Check sheet for the modelled part. Datum: model origin and axes. Units: mm. A direction names the side the tool comes from. Round coordinates to 2 decimals unless told otherwise and drop trailing zeros. Write each loop counter-clockwise with the first axis right and the second up, starting at its lowest first coordinate (ties: lowest second). Pieces come first, ordered by that corner, then holes. Notation, with made-up numbers: M -12,20 L -7,20 A30 ccw -7,56 Z; hole C 40,8 d8. An arc over 180 degrees is marked long. Answer in a Markdown table with one row per item.
```python
from build123d import *

# Parameters (mm, degrees)
SKETCH1_W           = 180
SKETCH1_H           = 140
BOSS_EXTRUDE1_DEPTH = 5.588
SKETCH3_R           = 2.65
CUT_EXTRUDE2_DEPTH  = 229.103541717
BOSS_EXTRUDE2_DEPTH = 5.588
SKETCH5_R           = 12.5
CUT_EXTRUDE3_DEPTH  = 246.465813799
SKETCH6_R           = 1.65
CUT_EXTRUDE4_DEPTH  = 246.465813799
SKETCH7_W           = 150
SKETCH7_H           = 42
BOSS_EXTRUDE3_DEPTH = 5.588
SKETCH2_R           = 2.15
CUT_EXTRUDE1_DEPTH  = 246.465813799
FILLET1_R           = 4


with BuildPart() as part:
    # Sketch1 → Boss-Extrude1 (new body)
    with BuildSketch(Plane(origin=(0, 0, 0), x_dir=(1, 0, 0), z_dir=(0, 1, 0))):
        with Locations((90, 70)):
            Rectangle(SKETCH1_W, SKETCH1_H)
    extrude(amount=BOSS_EXTRUDE1_DEPTH)

    # Sketch3 → Cut-Extrude2 (cut, through all)
    with BuildSketch(Plane(origin=(0, 5.588, 0), x_dir=(1, 0, 0), z_dir=(0, 1, 0))):
        with Locations(Location((90, 130, 0), (0, 0, 270))):
            Circle(SKETCH3_R)
        with Locations(Location((110, 130, 0), (0, 0, 270))):
            Circle(SKETCH3_R)
        with Locations(Location((130, 130, 0), (0, 0, 270))):
            Circle(SKETCH3_R)
        with Locations(Location((170, 130, 0), (0, 0, 270))):
            Circle(SKETCH3_R)
        with Locations(Location((30, 130, 0), (0, 0, 90))):
            Circle(SKETCH3_R)
        with Locations(Location((150, 130, 0), (0, 0, 270))):
            Circle(SKETCH3_R)
        with Locations(Location((10, 130, 0), (0, 0, 90))):
            Circle(SKETCH3_R)
        with Locations(Location((50, 130, 0), (0, 0, 90))):
            Circle(SKETCH3_R)
        with Locations(Location((70, 130, 0), (0, 0, 90))):
            Circle(SKETCH3_R)
        with Locations(Location((70, 10, 0), (0, 0, 270))):
            Circle(SKETCH3_R)
        with Locations(Location((50, 10, 0), (0, 0, 270))):
            Circle(SKETCH3_R)
        with Locations(Location((10, 10, 0), (0, 0, 270))):
            Circle(SKETCH3_R)
        with Locations(Location((150, 10, 0), (0, 0, 90))):
            Circle(SKETCH3_R)
        with Locations(Location((30, 10, 0), (0, 0, 270))):
            Circle(SKETCH3_R)
        with Locations(Location((170, 10, 0), (0, 0, 90))):
            Circle(SKETCH3_R)
        with Locations(Location((130, 10, 0), (0, 0, 90))):
            Circle(SKETCH3_R)
        with Locations(Location((110, 10, 0), (0, 0, 90))):
            Circle(SKETCH3_R)
        with Locations(Location((90, 10, 0), (0, 0, 90))):
            Circle(SKETCH3_R)
    extrude(amount=-CUT_EXTRUDE2_DEPTH, mode=Mode.SUBTRACT)

    # Sketch4 → Boss-Extrude2 (add, through all)
    with BuildSketch(Plane(origin=(0, 5.588, 0), x_dir=(1, 0, 0), z_dir=(0, 1, 0))):
        with BuildLine():
            Line((160, 140), (141.293647591, 140))
            ThreePointArc((141.293647591, 140), (135, 163.3), (128.706352409, 140))
            Line((128.706352409, 140), (110, 140))
            Line((110, 140), (110, 166.8))
            Line((110, 166.8), (160, 166.8))
            Line((160, 166.8), (160, 140))
        make_face()
    extrude(amount=-BOSS_EXTRUDE2_DEPTH)

    # Sketch5 → Cut-Extrude3 (cut, through all)
    with BuildSketch(Plane(origin=(0, 5.588, 0), x_dir=(1, 0, 0), z_dir=(0, 1, 0))):
        with Locations(Location((135, 150.8, 0), (0, 0, 270))):
            Circle(SKETCH5_R)
    extrude(amount=-CUT_EXTRUDE3_DEPTH, mode=Mode.SUBTRACT)

    # Sketch6 → Cut-Extrude4 (cut, through all)
    with BuildSketch(Plane(origin=(0, 5.588, 0), x_dir=(1, 0, 0), z_dir=(0, 1, 0))):
        with Locations(Location((115, 162.8, 0), (0, 0, 270))):
            Circle(SKETCH6_R)
        with Locations(Location((155, 162.8, 0), (0, 0, 270))):
            Circle(SKETCH6_R)
        with Locations(Location((155, 143.8, 0), (0, 0, 270))):
            Circle(SKETCH6_R)
        with Locations(Location((115, 143.8, 0), (0, 0, 270))):
            Circle(SKETCH6_R)
    extrude(amount=-CUT_EXTRUDE4_DEPTH, mode=Mode.SUBTRACT)

    # Sketch7 → Boss-Extrude3 (add, through all)
    with BuildSketch(Plane(origin=(0, 5.588, 0), x_dir=(1, 0, 0), z_dir=(0, 1, 0))):
        with Locations((-75, 70)):
            Rectangle(SKETCH7_W, SKETCH7_H)
    extrude(amount=-BOSS_EXTRUDE3_DEPTH)

    # Sketch2 → Cut-Extrude1 (cut, through all)
    with BuildSketch(Plane(origin=(0, 5.588, 0), x_dir=(1, 0, 0), z_dir=(0, 1, 0))):
        with Locations(Location((125, 81.5, 0), (0, 0, 270))):
            Circle(SKETCH2_R)
        with Locations(Location((125, 58.5, 0), (0, 0, 270))):
            Circle(SKETCH2_R)
        with Locations(Location((85, 81.5, 0), (0, 0, 270))):
            Circle(SKETCH2_R)
        with Locations(Location((165, 81.5, 0), (0, 0, 270))):
            Circle(SKETCH2_R)
        with Locations(Location((85, 58.5, 0), (0, 0, 270))):
            Circle(SKETCH2_R)
        with Locations(Location((165, 58.5, 0), (0, 0, 270))):
            Circle(SKETCH2_R)
        with Locations(Location((45, 81.5, 0), (0, 0, 270))):
            Circle(SKETCH2_R)
        with Locations(Location((45, 58.5, 0), (0, 0, 270))):
            Circle(SKETCH2_R)
        with Locations(Location((5, 81.5, 0), (0, 0, 270))):
            Circle(SKETCH2_R)
        with Locations(Location((5, 58.5, 0), (0, 0, 270))):
            Circle(SKETCH2_R)
        with Locations(Location((-35, 81.5, 0), (0, 0, 270))):
            Circle(SKETCH2_R)
        with Locations(Location((-35, 58.5, 0), (0, 0, 270))):
            Circle(SKETCH2_R)
        with Locations(Location((-75, 81.5, 0), (0, 0, 270))):
            Circle(SKETCH2_R)
        with Locations(Location((-75, 58.5, 0), (0, 0, 270))):
            Circle(SKETCH2_R)
        with Locations(Location((-115, 81.5, 0), (0, 0, 270))):
            Circle(SKETCH2_R)
        with Locations(Location((-115, 58.5, 0), (0, 0, 270))):
            Circle(SKETCH2_R)
        with Locations((-155, 81.5)):
            Circle(SKETCH2_R)
        with Locations((-155, 58.5)):
            Circle(SKETCH2_R)
    extrude(amount=-CUT_EXTRUDE1_DEPTH, mode=Mode.SUBTRACT)

    # Fillet1
    fillet1_edges = [part.edges().sort_by_distance(p)[0] for p in [
        (0, 2.794, -140),
        (0, 2.794, 0),
        (180, 2.794, 0),
        (180, 2.794, -140),
        (160, 2.794, -140),
        (160, 2.794, -166.8),
        (110, 2.794, -166.8),
        (110, 2.794, -140),
        (0, 2.794, -49),
        (-150, 2.794, -49),
        (-150, 2.794, -91),
        (0, 2.794, -91),
    ]]
    fillet(fillet1_edges, radius=FILLET1_R)


solid = part.part
```
1. Access from +Z, -Z, +X, -X, +Y, -Y to the whole of each face (thin tool, end or side, straight path). Record for faces 1 (the face through (170, 3, -140)), 2 (the face through (110, 3, -153)), 3 (the face through (0, 3, -24)).
Found:
| item | result |
|---|---|
| face 1 | -Z, +X, +Y, -Y |
| face 2 | -Z, -X, +Y, -Y |
| face 3 | +Z, -X, +Y, -Y |
2. Section check B-B, the plane y = 1.7. Count the separate pieces of the cut face and the enclosed holes in it, and give its area (3 significant figures).
Found:
| item | result |
|---|---|
| separate pieces | 1 |
| enclosed holes | 39 |
| area | 31,700 mm2 |
3. Section check D-D, the plane z = -100.5. Record the cut outline in (x, y), and give its area (3 significant figures).
Found:
| item | result |
|---|---|
| outline | M 0,0 L 180,0 L 180,5.59 L 0,5.59 Z |
| area | 1,010 mm2 |
4. Section check A-A, the plane z = -150.8. Record the cut outline in (x, y), and give its area (3 significant figures).
Found:
| item | result |
|---|---|
| outline | M 110,0 L 122.5,0 L 122.5,5.59 L 110,5.59 Z; M 147.5,0 L 160,0 L 160,5.59 L 147.5,5.59 Z |
| area | 140 mm2 |
5. Go/stop test with flat-tipped pins: pin 1 (3 mm diameter, centred on y = 3.5, z = -122, fed in from -X); pin 2 (6 mm diameter, centred on x = 3.5, z = -145.5, fed in from -Y); pin 3 (7 mm diameter, centred on x = -35, z = -81.5, fed in from +Y); pin 4 (1.5 mm diameter, centred on x = 55, y = 3.5, fed in from -Z). Record where each tip stops, or that it passes through.
Found:
| item | result |
|---|---|
| pin 1 | stops at x = 0 |
| pin 2 | passes through |
| pin 3 | stops at y = 5.59 |
| pin 4 | stops at z = -140 |
6. Section check C-C, the plane x = -124. Record the cut outline in (y, z).
Found:
| item | result |
|---|---|
| outline | M 0,-91 L 5.59,-91 L 5.59,-49 L 0,-49 Z |
7. Draft check along Z on faces 4 (the face through (147.394, 2.833, -152.427)), 5 (the face through (135, 3, -166.8)), 6 (the face through (89, 3, 0)). Enter one of: +Z half, -Z half, draft (parallel to the pull), parting line (faces both ways), or undercut.
Found:
| item | result |
|---|---|
| face 4 | undercut |
| face 5 | -Z half |
| face 6 | +Z half |
8. Scan lines: L1, parallel to Z at x = 165, y = 1.1; L2, parallel to X at y = 0.95, z = -123.5; L3, parallel to Z at x = -86, y = 4.6. Record each from-to range of solid material in increasing order.
Found:
| item | result |
|---|---|
| L1 | z = -140 to -83.65, -79.35 to -60.65, -56.35 to 0 |
| L2 | x = 0 to 180 |
| L3 | z = -91 to -49 |
